Geometry check sheet. Reference: the model listing, model coordinates, mm. A direction names the side the tool comes from. Give positions to 0.01 mm unless a question says otherwise; leave off trailing zeros. Loops run counter-clockwise (first coordinate to the right, second up) from the corner with the lowest first, then second, coordinate; pieces in that order, holes last. Notation, with made-up numbers: (10, -14) -> (24, -14) arc R21 cw to (24, 0) -> close; hole circle Ø8 at (22.5, 87.5). An arc over 180 degrees is marked (long way). Answer as a JSON object with one key per item and string values.
from build123d import *

# Parameters (mm, degrees)
F2_DEPTH = 25.4
F1_W     = 25.4
F1_H     = 50.8
F1_R     = 12.7
F3_DEPTH = 25.4


with BuildPart() as f2:
    # F0 (on Front) → F2 (new body)
    with BuildSketch(Plane.XZ):
        Polygon((0, 50.8), (0, 0), (50.8, 0), (50.8, 12.7), (42.995947, 12.7), (42.995947, 38.1), (50.8, 38.1), (50.8, 50.8), align=None)
    extrude(amount=-F2_DEPTH)

    # F1 (on Right) → F3 (join)
    with BuildSketch(Plane.YZ):
        with Locations((12.7, 25.4)):
            Rectangle(F1_W, F1_H)
        with BuildLine():
            Line((25.4, 50.8), (25.4, 0))
            Line((25.4, 0), (50.8, 0))
            ThreePointArc((50.8, 0), (68.760512, 7.439488), (76.2, 25.4))
            ThreePointArc((76.2, 25.4), (68.760512, 43.360512), (50.8, 50.8))
            Line((50.8, 50.8), (25.4, 50.8))
        make_face()
        with Locations((57.15, 28.366325)):
            Circle(F1_R, mode=Mode.SUBTRACT)
    extrude(amount=F3_DEPTH)


solid = f2.part
1) Section check B-B on z = 24.5. Record the cut outline in (x, y).
Geometry check:
{"outline": "(0, 0) -> (43, 0) -> (43, 25.4) -> (25.4, 25.4) -> (25.4, 45.05) -> (0, 45.05) -> close; (0, 69.25) -> (25.4, 69.25) -> (25.4, 76.18) -> (0, 76.18) -> close"}
2) Tool access check on faces 1 (the face through (47, 13, 38.1)), 2 (the face through (35, 25.4, 26)), 3 (the face through (0, 29, 26)). Record the directions out of +Z, -Z, +X, -X, +Y, -Y that give a thin tool (end or side, any length) a straight path to the whole face; none if there is none.
Geometry check:
{"face 1": "+X, +Y, -Y", "face 2": "+Z, -Z, +X, +Y", "face 3": "+Z, -Z, -X, +Y, -Y"}
3) Section check D-D on x = 22. Record the cut outline in (y, z).
Geometry check:
{"outline": "(0, 0) -> (50.8, 0) arc R25.4 ccw to (76.2, 25.4) arc R25.4 ccw to (50.8, 50.8) -> (0, 50.8) -> close; hole circle Ø25.4 at (57.15, 28.37)"}
4) Depth check by flat-ended pin: P1, Ø23, axis at y = 57.15, z = 28.37, coming from the -X side; P2, Ø7.5, axis at x = 38, z = 34.5, coming from the +Y side; P3, Ø6, axis at y = 37, z = 24.5, coming from the +X side; P4, Ø6, axis at x = 25, z = 42, coming from the +Y side. Enter the tip coordinate at first touch or a pass-through.
Geometry check:
{"P1": "passes through", "P2": "stops at y = 25.4", "P3": "stops at x = 25.4", "P4": "stops at y = 72.25"}
5) Section check A-A on y = 63. Record the cut outline in (x, z), plus the area to 3 significant figures.
Geometry check:
{"outline": "(0, 3.12) -> (25.4, 3.12) -> (25.4, 17.09) -> (0, 17.09) -> close; (0, 39.64) -> (25.4, 39.64) -> (25.4, 47.68) -> (0, 47.68) -> close", "area": "559 mm2"}
6) Material ranges on line 1 along Z through (x, y) = (45.5, 15); line 2 along X through (y, z) = (39, 18.5); line 3 along Y through (x, z) = (6, 23), recorded low to high. Write a range as from..to.
Geometry check:
{"line 1": "z = 0..12.7, 38.1..50.8", "line 2": "x = 0..25.4", "line 3": "y = 0..45.64, 68.66..76.09"}
7) Draft check along Z on faces 4 (the face through (47, 13, 12.7)), 5 (the face through (19, 19, 0)), 6 (the face through (25.4, 45, 20)), 7 (the face through (12.522, 44.462, 28.925)). Enter one of: pulls with the +Z half, pulls with the -Z half, needs draft (parallel to the pull), parting line crosses it, or undercut.
Geometry check:
{"face 4": "undercut", "face 5": "pulls with the -Z half", "face 6": "needs draft", "face 7": "undercut"}
8) Section check C-C on y = 30. Record the cut outline in (x, z).
Geometry check:
{"outline": "(0, 0) -> (25.4, 0) -> (25.4, 50.8) -> (0, 50.8) -> close"}
